Source: CAD feature listing. Evaluate the final solid. Frame: model axes, mm. Give positions to 0.01 mm unless a question says otherwise; leave off trailing zeros. Write each loop counter-clockwise with the first axis right and the second up, starting at its lowest first coordinate (ties: lowest second). Pieces come first, ordered by that corner, then holes. Notation, with made-up numbers: M -2.5,-1.75 L 12.5,-1.75 A23 ccw 12.5,22.25 Z; hole C -14,68 d6. An arc over 180 degrees is marked long. Use CSV: the item, a comma, the result in double quotes. Start each with the question number.
Autodesk Inventor part; units mm, degrees
ref_plane "YZ Plane" through (0, 0, 0) normal (1, 0, 0) x (0, 1, 0)
ref_plane "XZ Plane" through (0, 0, 0) normal (0, 1, 0) x (-1, 0, 0)
ref_plane "XY Plane" through (0, 0, 0) normal (0, 0, 1) x (1, 0, 0)
sketch "Sketch1" plane through (0, 0, 0) normal (0, 1, 0) x (-1, 0, 0)
  line L0 (0, 0) -> (-20.772, 0)
  line L1 (-20.772, 0) -> (-20.772, -9.19)
  line L2 (-20.772, -9.19) -> (0, -9.19)
  line L3 (0, -9.19) -> (0, 0)
  line L4 (-20.772, -9.19) -> (-30.572, -9.19)
  line L5 (-30.572, -9.19) -> (-30.572, 0)
  line L6 (-30.572, 0) -> (-20.772, 0)
  line L7 (-20.772, 0) -> (-20.772, -9.19)
  line L8 (-30.572, -9.19) -> (-51.344, -9.19)
  line L9 (-51.344, -9.19) -> (-51.344, 0)
  line L10 (-51.344, 0) -> (-30.572, 0)
  line L11 (-30.572, 0) -> (-30.572, -9.19)
  circle A0 centre (-5.772, -4.595) radius 1.75
  circle A1 centre (-15.772, -4.595) radius 1.75
  circle A2 centre (-35.572, -4.595) radius 1.75
  circle A3 centre (-45.572, -4.595) radius 1.75
  dimension "d0" = 20.772
  dimension "d1" = 9.19
  dimension "d2" = 9.8
  dimension "d3" = 9.19
  dimension "d4" = 20.772
  dimension "d5" = 9.19
  dimension "d6" = 3.5
  dimension "d7" = 3.5
  dimension "d8" = 3.5
  dimension "d9" = 3.5
  dimension "d10" = 5.772
  dimension "d11" = 10
  dimension "d12" = 5.772
  dimension "d13" = 10
extrude "Extrusion1" add sketch "Sketch1" along normal blind 4
chamfer "Chamfer1" distance 2.1825 angle 45 1 edges at (25.672, 4, -9.19)
chamfer "Chamfer2" distance 2.4 angle 45 4 edges at (7.522, 4, -4.595) (17.522, 4, -4.595) (37.322, 4, -4.595) (47.322, 4, -4.595)
equation "\"d12\" = d10"
equation "\"d13\" = d11"
properties part number "topSpacer"
Item 1: Section B-B (x = 26.5). Return the cut outline in (y, z), plus the area to 3 significant figures.
Item 2: Section C-C (y = 2.95). Return the cut outline in (x, z) (1 decimal).
Item 3: Contact query for flat-ended pins moving along their axis: pin 1 Ø1.5 at (x, z) = (45, -4) entering from -Y; pin 2 Ø5.5 at (x, z) = (15.772, -4.595) entering from +Y; pin 3 Ø1 at (x, z) = (37, -6) entering from +Y; pin 4 Ø2 at (x, z) = (5, -6.5) entering from -Y. Output: stop coordinate, or through.
Item 4: Section A-A (y = 0.9). Return the cut outline in (x, z) (3 decimals), plus the area to 3 significant figures.
Item 5: Pull-direction query (X, two-part tool) for faces 1 (the flat face through (0, 2, -5)), 2 (the flat face through (25.31, 2.68, -8.33)), 3 (the cylindrical face through (7.06, 0.79, -5.78)); classes: released by +X, released by -X, zero draft, split by the parting line, or undercut.
Item 6: Material intervals for probe 1 along X at (y, z) = (1.5, -4.25); probe 2 along X at (y, z) = (2, -5.25); probe 3 along Z at (x, y) = (47.5, 2.25), sorted ascending.
Output values:
1,outline,"M 0,-9.19 L 1.82,-9.19 L 4,-7.01 L 4,0 L 0,0 Z"
1,area,"34.4 mm2"
2,outline,"M 0,-8.1 L 51.3,-8.1 L 51.3,0 L 0,0 Z; hole C 5.8,-4.6 d6.2; hole C 15.8,-4.6 d6.2; hole C 35.6,-4.6 d6.2; hole C 45.6,-4.6 d6.2"
3,pin 1,"passes through"
3,pin 2,"stops at y = 2.6"
3,pin 3,"stops at y = 2.35"
3,pin 4,"stops at y = 0"
4,outline,"M 0,-9.19 L 51.344,-9.19 L 51.344,0 L 0,0 Z; hole C 5.772,-4.595 d3.5; hole C 15.772,-4.595 d3.5; hole C 35.572,-4.595 d3.5; hole C 45.572,-4.595 d3.5"
4,area,"433 mm2"
5,face 1,"released by -X"
5,face 2,"zero draft"
5,face 3,"undercut"
6,probe 1,"x = 0 to 4.06, 7.49 to 14.06, 17.49 to 33.86, 37.29 to 43.86, 47.29 to 51.34"
6,probe 2,"x = 0 to 3.72, 7.82 to 13.72, 17.82 to 33.52, 37.62 to 43.52, 47.62 to 51.34"
6,probe 3,"z = -8.76 to -6.02, -3.17 to 0"
